```python
from build123d import *

# Parameters (mm, degrees)
SKETCH1_W                 = 9.525
SKETCH1_H                 = 9.525
EXTRUDE1_DEPTH            = 40.64
SKETCH3_W                 = 9.525
SKETCH3_H                 = 8.89
EXTRUDE2_DEPTH            = 5.842
FILLET1_R                 = 6
SKETCH4_W                 = 9.525
SKETCH4_H                 = 12.7
EXTRUDE3_DEPTH            = 45
FILLET2_R                 = 3
F_6_CLEARANCE_HOLE1_D     = 3.7973
F_6_CLEARANCE_HOLE1_DEPTH = 9.906
F_6_CLEARANCE_HOLE1_TIP   = 1.140824014
F_6_CLEARANCE_HOLE3_D     = 3.7973
F_6_CLEARANCE_HOLE3_DEPTH = 24.892
F_6_CLEARANCE_HOLE3_TIP   = 1.140824014
F_6_CLEARANCE_HOLE4_D     = 3.7973
F_6_CLEARANCE_HOLE4_DEPTH = 29.972
F_6_CLEARANCE_HOLE4_TIP   = 1.140824014
FILLET3_R                 = 2


with BuildPart() as part:
    # Sketch1 → Extrude1 (new body)
    with BuildSketch(Plane.XY):
        with Locations((-4.7625, 4.7625)):
            Rectangle(SKETCH1_W, SKETCH1_H)
    extrude(amount=EXTRUDE1_DEPTH)

    # Sketch3 → Extrude2 (add)
    with BuildSketch(Plane.XZ):
        with Locations((-4.7625, 36.195)):
            Rectangle(SKETCH3_W, SKETCH3_H)
    extrude(amount=EXTRUDE2_DEPTH)

    # Fillet1
    fillet1_edges = [part.edges().sort_by_distance(p)[0] for p in [
        (-4.7625, -5.842, 40.64),
    ]]
    fillet(fillet1_edges, radius=FILLET1_R)

    # Sketch4 → Extrude3 (add)
    with BuildSketch(Plane.XZ):
        with Locations((-4.7625, 6.35)):
            Rectangle(SKETCH4_W, SKETCH4_H)
    extrude(amount=EXTRUDE3_DEPTH)

    # Fillet2
    fillet2_edges = [part.edges().sort_by_distance(p)[0] for p in [
        (-4.7625, 9.525, 0),
    ]]
    fillet(fillet2_edges, radius=FILLET2_R)

    # #6 Clearance Hole1
    with Locations(Plane(origin=(0, -3.175, 6.35), x_dir=(0, 0, 1), z_dir=(1, 0, 0))):
        with Locations((0, 0)):
            Hole(F_6_CLEARANCE_HOLE1_D / 2, depth=F_6_CLEARANCE_HOLE1_DEPTH)
            with Locations((0, 0, -(F_6_CLEARANCE_HOLE1_DEPTH + F_6_CLEARANCE_HOLE1_TIP / 2))):  # 118° drill point
                Cone(0, F_6_CLEARANCE_HOLE1_D / 2, F_6_CLEARANCE_HOLE1_TIP, mode=Mode.SUBTRACT)

    # #6 Clearance Hole3
    with Locations(Plane(origin=(-4.7625, -45, 6.35), x_dir=(-1, 0, 0), z_dir=(0, -1, 0))):
        with Locations((0, 0)):
            Hole(F_6_CLEARANCE_HOLE3_D / 2, depth=F_6_CLEARANCE_HOLE3_DEPTH)
            with Locations((0, 0, -(F_6_CLEARANCE_HOLE3_DEPTH + F_6_CLEARANCE_HOLE3_TIP / 2))):  # 118° drill point
                Cone(0, F_6_CLEARANCE_HOLE3_D / 2, F_6_CLEARANCE_HOLE3_TIP, mode=Mode.SUBTRACT)

    # #6 Clearance Hole4
    with Locations(Plane(origin=(-9.525, -24.68, 6.35), x_dir=(0, 0, -1), z_dir=(-1, 0, 0))):
        with Locations((0, 0)):
            Hole(F_6_CLEARANCE_HOLE4_D / 2, depth=F_6_CLEARANCE_HOLE4_DEPTH)
            with Locations((0, 0, -(F_6_CLEARANCE_HOLE4_DEPTH + F_6_CLEARANCE_HOLE4_TIP / 2))):  # 118° drill point
                Cone(0, F_6_CLEARANCE_HOLE4_D / 2, F_6_CLEARANCE_HOLE4_TIP, mode=Mode.SUBTRACT)

    # Fillet3
    fillet3_edges = [part.edges().sort_by_distance(p)[0] for p in [
        (-4.7625, -45, 12.7),
        (-4.7625, -45, 0),
    ]]
    fillet(fillet3_edges, radius=FILLET3_R)


solid = part.part
```
Input: part model. Units: mm. Frame: model coordinates. A direction names the side the tool comes from. Coordinates: 2 decimals unless noted, no trailing zeros. Loops run counter-clockwise (first coordinate to the right, second up) from the corner with the lowest first, then second, coordinate; pieces in that order, holes last. Notation, with made-up numbers: (0.5, -37) -> (5.5, -37) arc R11 cw to (5.5, -31) -> close; hole circle Ø4 at (83.25, -9.75). An arc over 180 degrees is marked (long way). Use a Markdown table: item, result.
1) Cut plane D-D (z = 33). Return the cut outline in (x, y) (3 decimals).
Results found:
| item | result |
|---|---|
| outline | (-9.525, -5.842) -> (0, -5.842) -> (0, 9.525) -> (-9.525, 9.525) -> close |
2) Cut plane C-C (z = 5.5). Give the number of separate pieces and of enclosed holes in the cut face, then the cut area to 3 significant figures.
Results found:
| item | result |
|---|---|
| separate pieces | 4 |
| enclosed holes | 0 |
| area | 380 mm2 |
3) Material intervals for line 1 along Y through (x, z) = (-8.25, 6.35) (3 decimals); line 2 along Z through (x, y) = (-2.15, -24.68); line 3 along Y through (x, z) = (-7, 5) (3 decimals), sorted ascending. Write a range as from..to.
Results found:
| item | result |
|---|---|
| line 1 | y = -45..-26.579, -22.781..-5.074, -1.276..9.525 |
| line 2 | z = 0..4.45, 8.25..12.7 |
| line 3 | y = -45..-26.015, -23.345..-4.51, -1.84..9.525 |
4) Access query for faces 1 (the cylindrical face through (-3.74, -21.85, 4.75)), 2 (the flat face through (0, -11, 11)), 3 (the flat face through (-5, -5.842, 33)), 4 (the flat face through (-5, 0, 22)). Directions: +Z, -Z, +X, -X, +Y, -Y. A direction counts if a zero-diameter tool reaches every point of the face in a straight line with its end or side. Return the directions, or none.
Results found:
| item | result |
|---|---|
| face 1 | -Y |
| face 2 | +Z, -Z, +X, +Y, -Y |
| face 3 | +Z, +X, -X, -Y |
| face 4 | +X, -X, -Y |
5) Cut plane A-A (y = -2). Return the cut outline in (x, z) (3 decimals), then the cut area to 3 significant figures.
Results found:
| item | result |
|---|---|
| outline | (-9.525, 0) -> (0, 0) -> (0, 4.859) -> (-9.525, 4.859) -> close; (-9.525, 7.841) -> (0, 7.841) -> (0, 12.7) -> (-9.525, 12.7) -> close; (-9.525, 31.75) -> (0, 31.75) -> (0, 40.238) -> (-9.525, 40.238) -> close |
| area | 173 mm2 |
6) Contact query for flat-ended pins moving along their axis: pin 1 (2.5 mm diameter, centred on y = -3.175, z = 6.35, fed in from -X); pin 2 (3 mm diameter, centred on x = -4.76, z = 6.35, fed in from -Y); pin 3 (3 mm diameter, centred on x = -6.5, y = -3.5, fed in from +Z); pin 4 (2.5 mm diameter, centred on x = -4.76, z = 6.35, fed in from -Y). Output: stop coordinate, or through.
Results found:
| item | result |
|---|---|
| pin 1 | passes through |
| pin 2 | stops at y = -19.87 |
| pin 3 | stops at z = 40.24 |
| pin 4 | stops at y = -19.72 |
7) Pull-direction query (Z, two-part tool) for faces 5 (the conical face through (-5.07, -19.17, 6.48)), 6 (the cylindrical face through (-4.696, 8.623, 0.855)), 7 (the cylindrical face through (-7.64, -24.763, 4.453)), 8 (the cylindrical face through (-4.696, -4.038, 38.929)); classes: released by +Z, released by -Z, zero draft, split by the parting line, or undercut.
Results found:
| item | result |
|---|---|
| face 5 | undercut |
| face 6 | released by -Z |
| face 7 | undercut |
| face 8 | released by +Z |
8) Cut plane B-B (x = -7.75). Return the cut outline in (y, z) (3 decimals).
Results found:
| item | result |
|---|---|
| outline | (-45, 2) arc R2 ccw to (-43, 0) -> (6.525, 0) arc R3 ccw to (9.525, 3) -> (9.525, 40.64) -> (0.158, 40.64) arc R6 ccw to (-5.842, 34.64) -> (-5.842, 31.75) -> (0, 31.75) -> (0, 12.7) -> (-43, 12.7) arc R2 ccw to (-45, 10.7) -> close; hole circle Ø3.797 at (-24.68, 6.35); hole circle Ø3.797 at (-3.175, 6.35) |
